Check sheet for the modelled part. Datum: model origin and axes. Units: mm. Face numbers are marked on the shaded views. A direction names the side the tool comes from. Give positions to 0.01 mm unless a question says otherwise; leave off trailing zeros. Order: outer loops, then holes, each group sorted by start corner. A loop starts at its lowest first (then second) coordinate and runs counter-clockwise, first axis right, second up. Notation, with made-up numbers: M 29,8 L 58,8 A18 cw 58,38 Z; hole C 11,42.25 d4. An arc over 180 degrees is marked long. Answer in a Markdown table with one row per item. Add a question column.
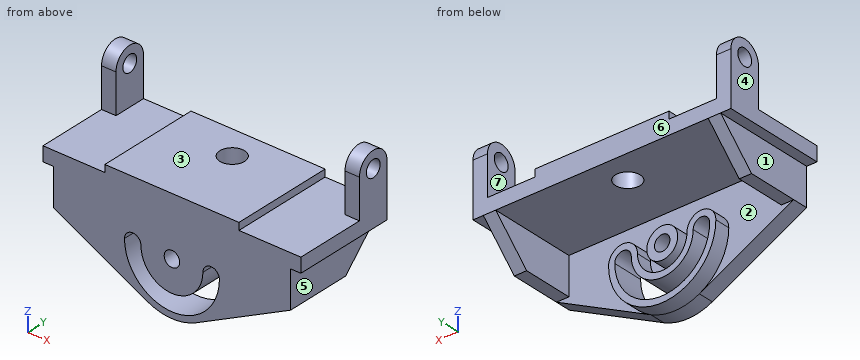
from build123d import *

# Parameters (mm, degrees)
SKETCH1_W           = 250
SKETCH1_H           = 100
BOSS_EXTRUDE1_DEPTH = 14
BOSS_EXTRUDE2_DEPTH = 100
SKETCH7_R           = 8
BOSS_EXTRUDE3_DEPTH = 14
SKETCH8_R           = 12
CUT_EXTRUDE1_DEPTH  = 25
BOSS_EXTRUDE4_DEPTH = 15
BOSS_EXTRUDE5_DEPTH = 12
SKETCH13_R          = 15
SKETCH13_R_2        = 7.5
BOSS_EXTRUDE6_DEPTH = 15
CUT_EXTRUDE2_START  = -15
SKETCH14_R          = 7.5
CUT_EXTRUDE2_DEPTH  = 15


with BuildPart() as part:
    # Sketch1 → Boss-Extrude1 (new body)
    with BuildSketch(Plane.XY):
        Rectangle(SKETCH1_W, SKETCH1_H)
    extrude(amount=BOSS_EXTRUDE1_DEPTH)

    # Sketch2 → Boss-Extrude2 (add)
    with BuildSketch(Plane(origin=(0, 50, 0), x_dir=(1, 0, 0), z_dir=(0, 1, 0))):
        Polygon((0, -14), (-65, -14), (-65, -21), (65, -21), (65, -14), align=None)
    extrude(amount=-BOSS_EXTRUDE2_DEPTH)

    # Sketch7 → Boss-Extrude3 (add)
    with BuildSketch(Plane.ZY.offset(125)):
        with BuildLine():
            Line((14, 50), (14, 18))
            Line((14, 18), (52, 18))
            ThreePointArc((52, 18), (68, 34), (52, 50))
            Line((52, 50), (14, 50))
        make_face()
        with Locations(Location((52, 34, 0), (0, 0, 270))):
            Circle(SKETCH7_R, mode=Mode.SUBTRACT)
    boss_extrude3 = extrude(amount=-BOSS_EXTRUDE3_DEPTH)

    # Mirror1: Boss-Extrude3 across plane
    add(boss_extrude3.mirror(Plane(origin=(0, 0, 0), x_dir=(0, 0, 1), z_dir=(1, 0, 0))))

    # Sketch8 → Cut-Extrude1 (cut)
    with BuildSketch(Plane(origin=(0, 0, 0), x_dir=(-1, 0, 0), z_dir=(0, 0, -1))):
        with Locations((0, 20)):
            Circle(SKETCH8_R)
    extrude(amount=-CUT_EXTRUDE1_DEPTH, mode=Mode.SUBTRACT)



with BuildPart() as body_2:
    # Sketch10 → Boss-Extrude4 (new body)
    with BuildSketch(Plane.XZ.offset(50)):
        with BuildLine():
            Line((115, 0), (115, -36))
            Line((115, -36), (23.513043478, -82.38034914))
            ThreePointArc((23.513043478, -82.38034914), (0, -88), (-23.513043478, -82.38034914))
            Line((-23.513043478, -82.38034914), (-115, -36))
            Line((-115, -36), (-115, 0))
            Line((-115, 0), (115, 0))
        make_face()
    extrude(amount=-BOSS_EXTRUDE4_DEPTH)


with BuildPart() as part_1:
    add(part.part)

    add(body_2.part)  # Boss-Extrude5 merges body 2
    # Sketch12 → Boss-Extrude5 (add)
    with BuildSketch(Plane(origin=(115, 0, 0), x_dir=(0, 0, -1), z_dir=(1, 0, 0))):
        Polygon((0, -35), (0, 50), (36, 14), (36, -35), align=None)
    boss_extrude5 = extrude(amount=-BOSS_EXTRUDE5_DEPTH)

    # Mirror2: Boss-Extrude5 across plane
    add(boss_extrude5.mirror(Plane(origin=(0, 0, 0), x_dir=(0, 0, 1), z_dir=(1, 0, 0))))

    # Sketch13 → Boss-Extrude6 (add)
    # profile 1 of 2: a face of its own
    with BuildSketch(Plane(origin=(0, -35, 0), x_dir=(1, 0, 0), z_dir=(0, 1, 0))):
        with Locations((0, 36)):
            Circle(SKETCH13_R)
        with Locations(Location((0, 36, 0), (0, 0, 180))):
            Circle(SKETCH13_R_2, mode=Mode.SUBTRACT)
    # profile 2 of 2: a face of its own
    with BuildSketch(Plane(origin=(0, -35, 0), x_dir=(1, 0, 0), z_dir=(0, 1, 0))):
        with BuildLine():
            ThreePointArc((24, 36), (0, 60), (-24, 36))
            ThreePointArc((-24, 36), (-38, 22), (-52, 36))
            ThreePointArc((-52, 36), (0, 88), (52, 36))
            ThreePointArc((52, 36), (38, 22), (24, 36))
        make_face()
        with BuildLine():
            ThreePointArc((30, 36), (0, 66), (-30, 36))
            ThreePointArc((-30, 36), (-38, 28), (-46, 36))
            ThreePointArc((-46, 36), (0, 82), (46, 36))
            ThreePointArc((46, 36), (38, 28), (30, 36))
        make_face(mode=Mode.SUBTRACT)
    extrude(amount=BOSS_EXTRUDE6_DEPTH)

    # Sketch14 → Cut-Extrude2 (cut)
    with BuildSketch(Plane(origin=(0, -35, 0), x_dir=(1, 0, 0), z_dir=(0, 1, 0)).offset(CUT_EXTRUDE2_START)):
        with Locations(Location((0, 36, 0), (0, 0, 180))):
            Circle(SKETCH14_R)
        with BuildLine():
            ThreePointArc((30, 36), (0, 66), (-30, 36))
            ThreePointArc((-30, 36), (-38, 28), (-46, 36))
            ThreePointArc((-46, 36), (0, 82), (46, 36))
            ThreePointArc((46, 36), (38, 28), (30, 36))
        make_face()
    extrude(amount=CUT_EXTRUDE2_DEPTH, mode=Mode.SUBTRACT)


solid = part_1.part
Q1. Draft check along X on the marked faces 4, 5, 6 and 7. Enter one of: pulls with the +X half, pulls with the -X half, needs draft (parallel to the pull), parting line crosses it, or undercut.
Q2. Cross-section at C-C (y = -32). Record the boundary of the cut face in (x, z).
Q3. Cross-section at B-B (z = 29). Record the boundary of the cut face in (x, y), and give its area (3 significant figures).
Q4. Cross-section at A-A (x = 0). Record the boundary of the cut face in (y, z), and give its area (3 significant figures).
Q5. Tool access check on the marked faces 1, 2 and 3. Record the directions out of +Z, -Z, +X, -X, +Y, -Y that give a thin tool (end or side, any length) a straight path to the whole face; none if there is none.
Q6. Go/stop test with flat-tipped pins: pin 1 (8 mm diameter, centred on x = -98.5, y = -16.5, fed in from -Z); pin 2 (1.5 mm diameter, centred on x = 41, y = -12, fed in from +Z); pin 3 (2 mm diameter, centred on y = 23.5, z = -13.5, fed in from -X); pin 4 (2 mm diameter, centred on x = -97.5, z = -47, fed in from -Y) (3 decimals). Record where each tip stops, or that it passes through.
Q7. Thickness scan on probe 1 along Z at (x, y) = (0, -26.25); probe 2 along Z at (x, y) = (-115.75, 34); probe 3 along Y at (x, z) = (0, 12.75). Record the ranges inside material, lowest first.
Q8. Cross-section at D-D (x = -38.5). Record the boundary of the cut face in (y, z).
Values follow:
| question | item | result |
|---|---|---|
| 1 | face 4 | pulls with the -X half |
| 1 | face 5 | pulls with the +X half |
| 1 | face 6 | needs draft |
| 1 | face 7 | undercut |
| 2 | outline | M -125,0 L -115,0 L -115,-36 L -103,-36 L -103,0 L 103,0 L 103,-36 L 115,-36 L 115,0 L 125,0 L 125,14 L 65,14 L 65,21 L -65,21 L -65,14 L -125,14 Z; M -52,-36 A52 ccw 52,-36 A14 ccw 24,-36 A24 cw -24,-36 A14 ccw Z; C 0,-36 d30; hole M -46,-36 A46 ccw 46,-36 A8 ccw 30,-36 A30 cw -30,-36 A8 ccw Z; hole C 0,-36 d15 |
| 3 | outline | M -125,18 L -111,18 L -111,50 L -125,50 Z; M 111,18 L 125,18 L 125,50 L 111,50 Z |
| 3 | area | 896 mm² |
| 4 | outline | M -50,-88 L -20,-88 L -20,-82 L -50,-82 Z; M -50,-66 L -20,-66 L -20,-60 L -35,-60 L -35,-51 L -20,-51 L -20,-43.5 L -50,-43.5 Z; M -50,-28.5 L -20,-28.5 L -20,-21 L -35,-21 L -35,0 L 8,0 L 8,21 L -50,21 Z; M 32,0 L 50,0 L 50,21 L 32,21 Z |
| 4 | area | 2,860 mm² |
| 5 | face 1 | -Z, -X, +Y, -Y |
| 5 | face 2 | +Y |
| 5 | face 3 | +Z, +Y, -Y |
| 6 | pin 1 | z = 0 |
| 6 | pin 2 | z = 21 |
| 6 | pin 3 | x = -115 |
| 6 | pin 4 | through |
| 7 | probe 1 | -88 to -82, -66 to -60, -51 to -43.5, -28.5 to -21, 0 to 21 |
| 7 | probe 2 | 0 to 44, 60 to 68 |
| 7 | probe 3 | -50 to 8, 32 to 50 |
| 8 | outline | M -50,-74.78 L -35,-74.78 L -35,-70.95 L -20,-70.95 L -20,-61.17 L -50,-61.17 Z; M -50,-28.02 L -20,-28.02 L -20,-22.01 L -35,-22.01 L -35,0 L 50,0 L 50,21 L -50,21 Z |
